Study the drawing (mm; zero at the part's minimum x, y, z) and answer. A direction names the side the tool comes from. Coordinates: 2 decimals unless noted, no trailing zeros. Order: outer loops, then holes, each group sorted by start corner. A loop starts at its lowest first (then second) coordinate and runs counter-clockwise, first axis right, second up. Notation, with made-up numbers: (16.5, 15.25) -> (42.5, 15.25) arc R20 cw to (42.5, 33.25) -> close; hole circle Ø9 at (-22.5, 43.25). An arc over 180 degrees is marked (long way). One line per question, with ' | ' between items.
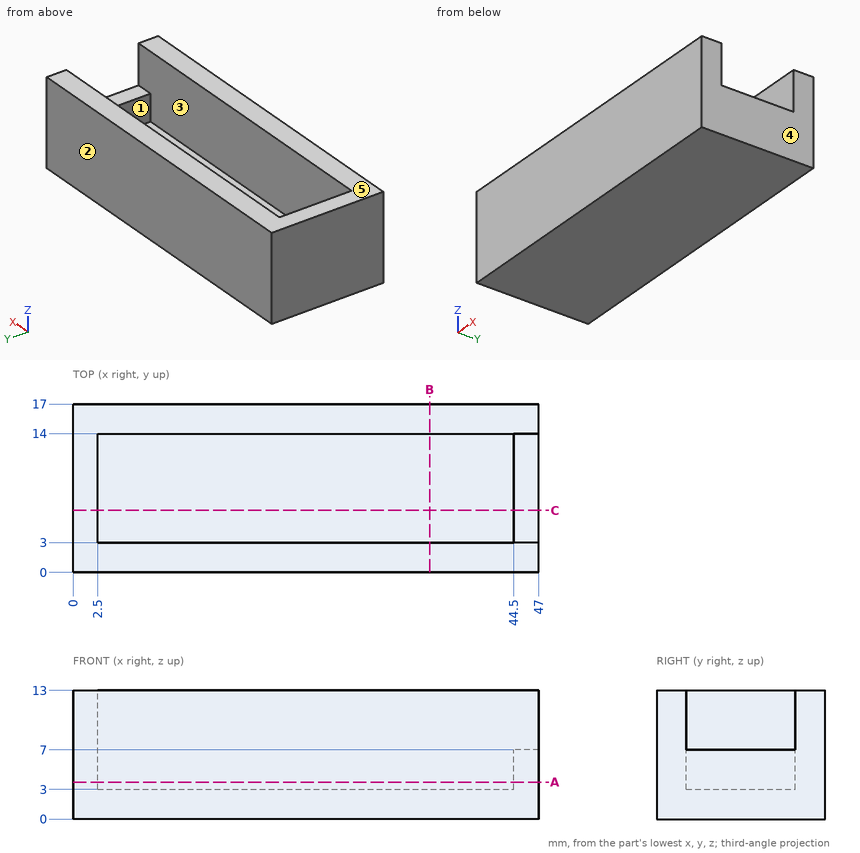
Item 1: Section A-A, the plane z = 3.75 is taken. Give the vertices of the cut face in (x, y).
Computed values:
outline: (0, 0) -> (47, 0) -> (47, 17) -> (0, 17) -> close; hole (2.5, 3) -> (44.5, 3) -> (44.5, 14) -> (2.5, 14) -> close
Item 2: Determine the mould class of the marked faces 3, 4 and 5 for opening direction X: pulls with the +X half, pulls with the -X half, needs draft (parallel to the pull), parting line crosses it, or undercut.
Computed values:
face 3: undercut | face 4: pulls with the +X half | face 5: needs draft
Item 3: Section B-B, the plane x = 36 is taken. Give the vertices of the cut face in (y, z), plus the area to 3 significant figures.
Computed values:
outline: (0, 0) -> (17, 0) -> (17, 13) -> (14, 13) -> (14, 3) -> (3, 3) -> (3, 13) -> (0, 13) -> close | area: 111 mm^2
Item 4: For the marked faces 1 and 2, determine the directions among +Z, -Z, +X, -X, +Y, -Y from which every point of the face is accessible in a straight line to the end or side of a thin tool.
Computed values:
face 1: +Z | face 2: +Z, -Z, +X, -X, +Y
Item 5: Section C-C, the plane y = 6.25 is taken. Give the vertices of the cut face in (x, z).
Computed values:
outline: (0, 0) -> (47, 0) -> (47, 7) -> (44.5, 7) -> (44.5, 3) -> (2.5, 3) -> (2.5, 13) -> (0, 13) -> close
Item 6: Each of these flat-tipped pins is pushed along its axis until it touches: pin 1 Ø1.2 at (x, y) = (46, 8) entering from +Z; pin 2 Ø5.5 at (x, y) = (25.5, 6) entering from +Z. Where does it stop, or does it pass through?
Computed values:
pin 1: stops at z = 7 | pin 2: stops at z = 3
Item 7: Find the intervals of material crossed by L1, parallel to Y at x = 31, z = 10.5; L2, parallel to X at y = 4.75, z = 4; L3, parallel to X at y = 8.5, z = 12, in increasing order.
Computed values:
L1: y = 0 to 3, 14 to 17 | L2: x = 0 to 2.5, 44.5 to 47 | L3: x = 0 to 2.5
